Input: part model. Units: mm. Frame: model coordinates. A direction names the side the tool comes from. Round coordinates to 2 decimals unless told otherwise and drop trailing zeros. Loops run counter-clockwise (first coordinate to the right, second up) from the corner with the lowest first, then second, coordinate; pieces in that order, holes last. Notation, with made-up numbers: (2.25, 45) - (21.25, 45) arc R27 cw to (21.25, 66) - close; hole circle Ø1 at (81, 78.25). An arc over 180 degrees is marked (long way). One line per question, with ' | ' between items. Start each with the question number.
Item 1: First-contact query: pin 1 (0.9 mm diameter, centred on x = 10, y = 2, fed in from +Z); pin 2 (1.8 mm diameter, centred on x = 30, z = 0, fed in from -Y). Flat tips, straight axial feed; report the tip coordinate or a pass-through.
Item 2: Material intervals for line 1 along X through (y, z) = (2.35, 0); line 2 along Z through (x, y) = (30, 1.75); line 3 along Z through (x, y) = (15.5, 1), sorted ascending.
Item 3: Set-up query: faces 4 (the face through (15, 1, 3)), 5 (the face through (-1.5, 1.48, -0.07)). Return all of +Z, -Z, +X, -X, +Y, -Y with unobstructed straight access to the full face (end or side cutting, diameter ignored); none if empty.
Item 4: Section C-C, the plane y = 0.5. Return loops of the section in (x, z), plus the area to 3 significant figures.
Item 5: Section D-D, the plane x = 22. Return loops of the section in (y, z).
Item 6: Draft query along X for faces 1 (the face through (-5.496, 1.479, -0.197)), 2 (the face through (15, 3, 0)), 3 (the face through (15, 1, -3)). Return one class per face: pulls with the +X half, pulls with the -X half, needs draft (parallel to the pull), parting line crosses it, or undercut.
Item 7: Section B-B, the plane x = 0. Return loops of the section in (y, z).
Item 8: Section A-A, the plane z = 0. Return loops of the section in (x, y).
```python
from build123d import *

# Parameters (mm, degrees)
SKETCH1_R           = 1.5
BOSS_EXTRUDE1_DEPTH = 3


with BuildPart() as part:
    # Sketch1 → Boss-Extrude1 (new body)
    with BuildSketch(Plane(origin=(0, 0, 0), x_dir=(1, 0, 0), z_dir=(0, 1, 0))):
        with BuildLine():
            ThreePointArc((4.609772229, 3), (-5.5, 0), (4.609772229, -3))
            Line((4.609772229, -3), (25.390227771, -3))
            ThreePointArc((25.390227771, -3), (35.5, 0), (25.390227771, 3))
            Line((25.390227771, 3), (4.609772229, 3))
        make_face()
        Circle(SKETCH1_R, mode=Mode.SUBTRACT)
        with Locations((30, 0)):
            Circle(SKETCH1_R, mode=Mode.SUBTRACT)
    extrude(amount=BOSS_EXTRUDE1_DEPTH)


solid = part.part
```
Return value:
1) pin 1: z = 3 | pin 2: through
2) line 1: -5.5 to -1.5, 1.5 to 28.5, 31.5 to 35.5 | line 2: -5.5 to -1.5, 1.5 to 5.5 | line 3: -3 to 3
3) face 4: +Z, +Y, -Y | face 5: +Y, -Y
4) outline: (4.61, -3) - (25.39, -3) arc R5.5 ccw (long way) to (25.39, 3) - (4.61, 3) arc R5.5 ccw (long way) to start; hole circle Ø3 at (0, 0); hole circle Ø3 at (30, 0) | area: 293 mm2
5) outline: (0, -3) - (3, -3) - (3, 3) - (0, 3) - close
6) face 1: undercut | face 2: needs draft | face 3: undercut
7) outline: (0, -5.5) - (3, -5.5) - (3, -1.5) - (0, -1.5) - close; (0, 1.5) - (3, 1.5) - (3, 5.5) - (0, 5.5) - close
8) outline: (-5.5, 0) - (-1.5, 0) - (-1.5, 3) - (-5.5, 3) - close; (1.5, 0) - (28.5, 0) - (28.5, 3) - (1.5, 3) - close; (31.5, 0) - (35.5, 0) - (35.5, 3) - (31.5, 3) - close
